For this review, use the dimensioned drawing (mm, ordinates from the lowest corner) and the shaded views. A direction names the side the tool comes from. Round coordinates to 2 decimals unless told otherwise and drop trailing zeros. Order: outer loops, then holes, each group sorted by start corner. A loop starts at its lowest first (then second) coordinate and runs counter-clockwise, first axis right, second up. Notation, with made-up numbers: (53, 30.5) -> (107, 30.5) arc R6 cw to (107, 36.5) -> close; hole circle Ø3 at (-12, -30.5). An arc over 180 degrees is marked (long way). Answer in a Markdown table with one row per item.
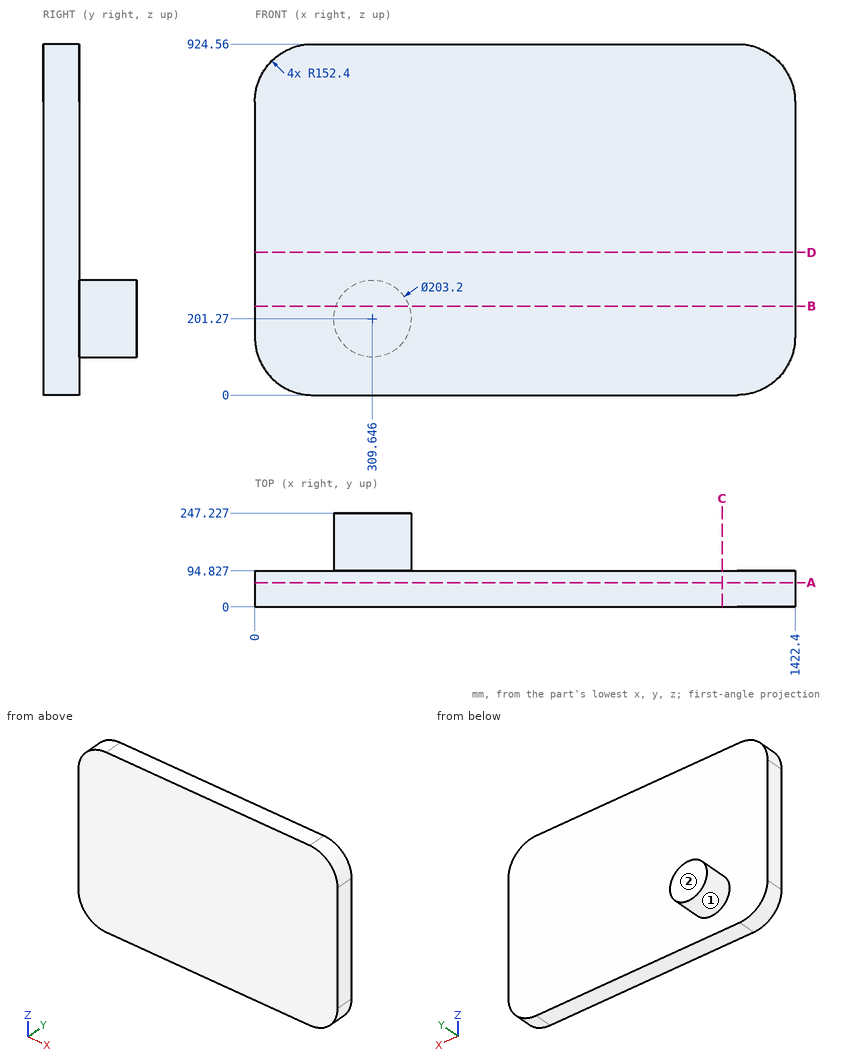
Q1. Tool access review of the marked faces 1 and 2: name each direction out of +Z, -Z, +X, -X, +Y, -Y from which nothing blocks a thin tool from reaching the whole face with its end or side.
Answer key:
| item | result |
|---|---|
| face 1 | +Y |
| face 2 | +Z, -Z, +X, -X, +Y |
Q2. Take a section at D-D, the plane z = 375.5. Write out the cut boundary in (x, y).
Answer key:
| item | result |
|---|---|
| outline | (0, 0) -> (1422.4, 0) -> (1422.4, 94.83) -> (0, 94.83) -> close |
Q3. Take a section at A-A, the plane y = 64. Write out the cut boundary in (x, z), then the cut area to 3 significant figures.
Answer key:
| item | result |
|---|---|
| outline | (0, 152.4) arc R152.4 ccw to (152.4, 0) -> (1270, 0) arc R152.4 ccw to (1422.4, 152.4) -> (1422.4, 772.16) arc R152.4 ccw to (1270, 924.56) -> (152.4, 924.56) arc R152.4 ccw to (0, 772.16) -> close |
| area | 1,300,000 mm^2 |
Q4. To check wall thickness, follow probe 1 along Y at (x, z) = (1314, 111); probe 2 along X at (y, z) = (190, 145); probe 3 along X at (y, z) = (170, 207.5) (1 decimal). State the ranges of each line that lie inside material, in increasing order.
Answer key:
| item | result |
|---|---|
| probe 1 | y = 0 to 94.83 |
| probe 2 | x = 225.05 to 394.24 |
| probe 3 | x = 208.2 to 411.1 |
Q5. Clearance check with a flat-ended pin moving along its axis: pin 1 Ø2 at (x, z) = (464.5, 727) entering from +Y. State where the tip first meets the part, or that it passes through.
Answer key:
| item | result |
|---|---|
| pin 1 | stops at y = 94.83 |
Q6. Take a section at C-C, the plane x = 1230.5. Write out the cut boundary in (y, z).
Answer key:
| item | result |
|---|---|
| outline | (0, 0) -> (94.83, 0) -> (94.83, 924.56) -> (0, 924.56) -> close |
Q7. Take a section at B-B, the plane z = 234. Write out the cut boundary in (x, y).
Answer key:
| item | result |
|---|---|
| outline | (0, 0) -> (1422.4, 0) -> (1422.4, 94.83) -> (405.83, 94.83) -> (405.83, 247.23) -> (213.46, 247.23) -> (213.46, 94.83) -> (0, 94.83) -> close |
